The drawing under review shows one solid part. Ordinate dimensions are in mm from its lowest x, y, z. A direction names the side the tool comes from. Round coordinates to 2 decimals unless told otherwise and drop trailing zeros. Order: outer loops, then holes, each group sorted by start corner. A loop starts at its lowest first (then second) coordinate and runs counter-clockwise, first axis right, second up. Notation, with made-up numbers: M 52,-5 L 58,-5 A33 ccw 58,34 Z; hole C 27,44 d7. An arc over 180 degrees is marked long. Answer as a JSON object with one key per item and string values.
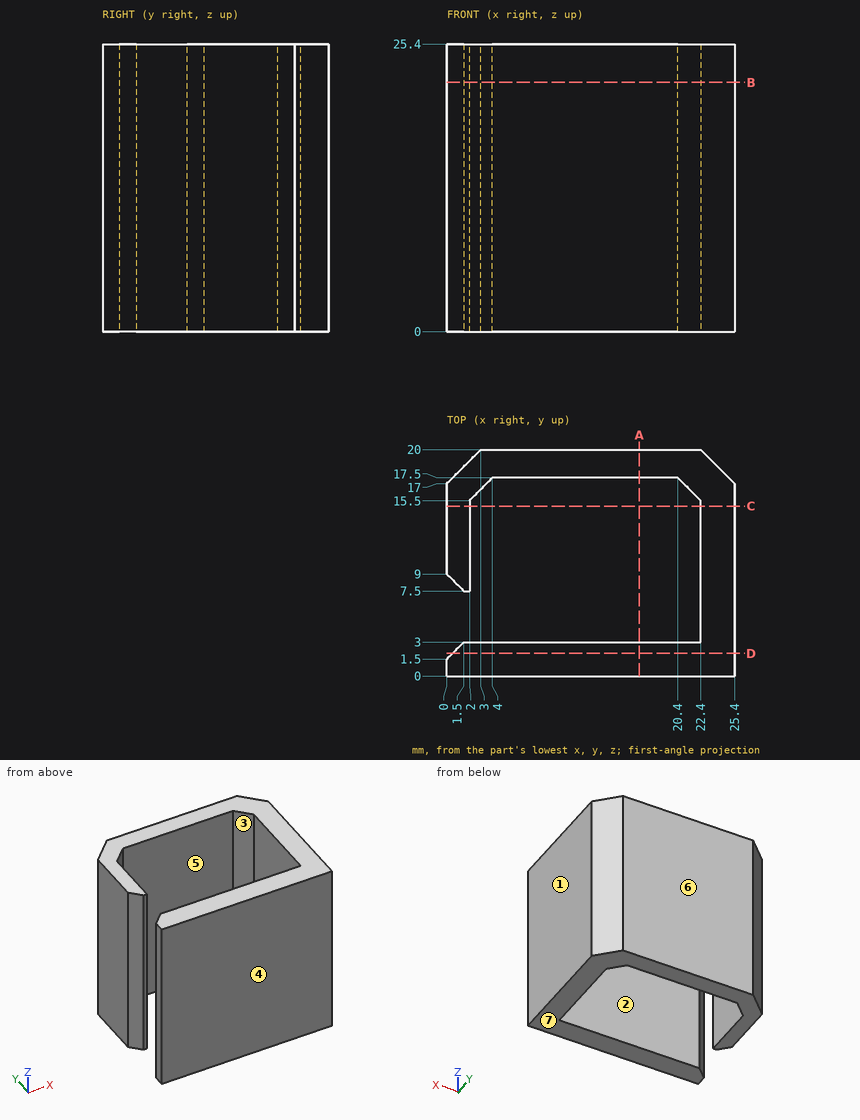
1) Machinability: for the marked faces 1, 2 and 3, which of the approach directions +Z, -Z, +X, -X, +Y, -Y give a long, thin tool a straight path to every point of the face, cutting with its end or side? Answer none if there is none.
Geometry check:
{"face 1": "+Z, -Z, +X, +Y, -Y", "face 2": "+Z, -Z, -X", "face 3": "+Z, -Z"}
2) For L1, parallel to Y at x = 6.5, z = 19; L2, parallel to X at y = 12.5, z = 21.5; L3, parallel to X at y = 6, z = 12.5, list the stretches that pass through material, from the lowest coordinate up.
Geometry check:
{"L1": "y = 0 to 3, 17.5 to 20", "L2": "x = 0 to 2, 22.4 to 25.4", "L3": "x = 22.4 to 25.4"}
3) Insertion check: P1, Ø8, axis at x = 11, z = 16.5, coming from the -Y side. The pin has a flat end and moves straight along its axis. Give the tip position at first contact, or say it passes through.
Geometry check:
{"P1": "stops at y = 0"}
4) Add section C-C on y = 15. State the section outline as (x, z) points.
Geometry check:
{"outline": "M 0,0 L 2,0 L 2,25.4 L 0,25.4 Z; M 22.4,0 L 25.4,0 L 25.4,25.4 L 22.4,25.4 Z"}
5) Mouldability with a two-part tool opening along Y and no side actions: class the marked faces 4, 5, 6 and 7 as +Y half, -Y half, draft (parallel to the pull), parting line (faces both ways), or undercut.
Geometry check:
{"face 4": "-Y half", "face 5": "undercut", "face 6": "+Y half", "face 7": "draft"}
6) Add section D-D on y = 2. State the section outline as (x, z) points.
Geometry check:
{"outline": "M 0.5,0 L 25.4,0 L 25.4,25.4 L 0.5,25.4 Z"}
7) Add section B-B on z = 22. State the section outline as (x, y) points, and give its area (3 significant figures).
Geometry check:
{"outline": "M 0,0 L 25.4,0 L 25.4,17 L 22.4,20 L 3,20 L 0,17 L 0,9 L 1.5,7.5 L 2,7.5 L 2,15.5 L 4,17.5 L 20.4,17.5 L 22.4,15.5 L 22.4,3 L 1.5,3 L 0,1.5 Z", "area": "196 mm²"}
8) Add section A-A on x = 17. State the section outline as (y, z) points.
Geometry check:
{"outline": "M 0,0 L 3,0 L 3,25.4 L 0,25.4 Z; M 17.5,0 L 20,0 L 20,25.4 L 17.5,25.4 Z"}
